```python
from build123d import *

# Parameters (mm, degrees)
SKETCH1_W               = 1200
SKETCH1_H               = 1500
BOSS_EXTRUDE1_DEPTH     = 160
BOSS_EXTRUDE2_DEPTH     = 1270
SKETCH3_W               = 125
SKETCH3_H               = 1120
CUT_EXTRUDE2_DEPTH      = 30
LPATTERN1_COUNT         = 6
LPATTERN1_PITCH         = 165
SKETCH4_W               = 125
SKETCH4_H               = 1120
CUT_EXTRUDE3_DEPTH      = 30
LPATTERN2_COUNT         = 6
LPATTERN2_PITCH         = 165
CUT_EXTRUDE5_DEPTH      = 70
CUT_EXTRUDE5_DEPTH_BACK = 3200
SKETCH5_W               = 160
SKETCH5_H               = 1200
BOSS_EXTRUDE3_DEPTH     = 40
CUT_EXTRUDE6_DEPTH      = 1622
SKETCH8_R               = 25
BOSS_EXTRUDE4_DEPTH     = 284.986135381
SKETCH10_R              = 25
BOSS_EXTRUDE5_DEPTH     = 408.541682101


with BuildPart() as part:
    # Sketch1 → Boss-Extrude1 (new body)
    with BuildSketch(Plane(origin=(0, 0, 0), x_dir=(0, 0, -1), z_dir=(1, 0, 0))):
        with Locations((564.361948956, -723.13225058)):
            Rectangle(SKETCH1_W, SKETCH1_H)
    extrude(amount=BOSS_EXTRUDE1_DEPTH)

    # Sketch2 → Boss-Extrude2 (add)
    with BuildSketch(Plane.ZY):
        Polygon((293.387128793, -77.723630642), (-775.820700233, 467.064969046), (-789.440415225, 440.33477332), (279.767413801, -104.453826367), align=None)
        Polygon((333.138052406, -383.823490794), (-736.06977662, -928.612090481), (-722.450061628, -955.342286207), (346.757767398, -410.553686519), align=None)
    extrude(amount=BOSS_EXTRUDE2_DEPTH)

    # Sketch3 → Cut-Extrude2 (cut)
    with BuildSketch(Plane(origin=(0, -466.202007743, 237.541787551), x_dir=(-1, 0, 0), z_dir=(0, -0.8910065241883673, 0.45399049973954775))):
        with Locations((1167.066310977, 477.424040248)):
            Rectangle(SKETCH3_W, SKETCH3_H)
    cut_extrude2 = extrude(amount=-CUT_EXTRUDE2_DEPTH, mode=Mode.SUBTRACT)

    # LPattern1: Cut-Extrude2 ×6
    with Locations(*[(i * LPATTERN1_PITCH, 0, 0) for i in range(1, LPATTERN1_COUNT)]):
        add(cut_extrude2, mode=Mode.SUBTRACT)

    # Sketch4 → Cut-Extrude3 (cut)
    with BuildSketch(Plane(origin=(0, 30.243173593, 15.409666619), x_dir=(-1, 0, 0), z_dir=(0, -0.891006524188367, -0.4539904997395487))):
        with Locations((1167.5, 303.304364216)):
            Rectangle(SKETCH4_W, SKETCH4_H)
    cut_extrude3 = extrude(amount=-CUT_EXTRUDE3_DEPTH, mode=Mode.SUBTRACT)

    # LPattern2: Cut-Extrude3 ×6
    with Locations(*[(i * LPATTERN2_PITCH, 0, 0) for i in range(1, LPATTERN2_COUNT)]):
        add(cut_extrude3, mode=Mode.SUBTRACT)

    # Sketch5 → Cut-Extrude5 (cut, two sides: drawn at the far end of the back side and taken through both)
    with BuildSketch(Plane(origin=(0, 26.86774942, 0), x_dir=(1, 0, 0), z_dir=(0, 1, 0)).offset(-CUT_EXTRUDE5_DEPTH_BACK)):
        with Locations((80, 564.361948956)):
            Rectangle(SKETCH5_W, SKETCH5_H)
    extrude(amount=CUT_EXTRUDE5_DEPTH + CUT_EXTRUDE5_DEPTH_BACK, mode=Mode.SUBTRACT)


with BuildPart() as cut_extrude5_piece_1:
    # of the separate pieces the step leaves, piece 1, a body of its own (cut_extrude5_pieces)
    add(part.part.solids().sort_by_distance((0, -104.453826367, 279.767413801))[0])



with BuildPart() as cut_extrude5_piece_2:
    # of the separate pieces the step leaves, piece 2, a body of its own (cut_extrude5_pieces)
    add(part.part.solids().sort_by_distance((0, -410.553686519, 346.757767398))[0])


with BuildPart() as cut_extrude5_piece_1_1:
    add(cut_extrude5_piece_1.part)

    add(cut_extrude5_piece_2.part)  # Boss-Extrude3 merges Cut-Extrude5 piece 2
    # Sketch6 → Boss-Extrude3 (add)
    with BuildSketch(Plane(origin=(0, 0, 0), x_dir=(0, 0, -1), z_dir=(1, 0, 0))):
        Polygon((-293.387128793, -77.723630642), (-346.757767398, -410.553686519), (722.450061628, -955.342286207), (775.820700233, 467.064969046), align=None)
    extrude(amount=BOSS_EXTRUDE3_DEPTH)

    # Sketch7 → Cut-Extrude6 (cut)
    with BuildSketch(Plane(origin=(40, 0, 0), x_dir=(0, 0, -1), z_dir=(1, 0, 0))):
        Polygon((779.00615654, 352.336895643), (771.36995873, 348.446058521), (722.450061628, -955.342286207), (-346.757767398, -410.553686519), (-313.704524727, -204.427005397), (-484.232359842, -291.315277235), (-228.557425004, -1565.861378417), (1566.457503136, -862.127788671), align=None)
        Polygon((771.36995873, 348.446058521), (-13.619714992, -51.52615783), (-313.704524727, -204.427005397), (-346.757767398, -410.553686519), (722.450061628, -955.342286207), align=None)
    extrude(amount=-CUT_EXTRUDE6_DEPTH, mode=Mode.SUBTRACT)

    # Sketch8 → Boss-Extrude4 (add)
    with BuildSketch(Plane(origin=(40, 0, 0), x_dir=(0, 0, -1), z_dir=(1, 0, 0))):
        with Locations(Location((-198.070529097, -84.596305771, 0), (0, 0, 180))):
            Circle(SKETCH8_R)
        with Locations(Location((678.163657159, 359.269351402, 0), (0, 0, 180))):
            Circle(SKETCH8_R)
    extrude(amount=BOSS_EXTRUDE4_DEPTH)

    # Sketch10 → Boss-Extrude5 (add)
    with BuildSketch(Plane.ZY.offset(1270)):
        with Locations(Location((-716.617969304, 403.229883829, 0), (0, 0, 153))):
            Circle(SKETCH10_R)
        with Locations(Location((171.176211965, -49.123845441, 0), (0, 0, 153))):
            Circle(SKETCH10_R)
    extrude(amount=BOSS_EXTRUDE5_DEPTH)


solid = cut_extrude5_piece_1_1.part
```
Model file for the job. Use its own axes, mm. A direction names the side the tool comes from. Coordinates: 2 decimals unless noted, no trailing zeros. Order: outer loops, then holes, each group sorted by start corner. A loop starts at its lowest first (then second) coordinate and runs counter-clockwise, first axis right, second up. Notation, with made-up numbers: (77.25, 82) - (132.25, 82) arc R8 cw to (132.25, 95) - close; hole circle Ø6 at (42, 55.5). An arc over 180 degrees is marked (long way). Return JSON: item names as keys, results as strings. Group by question number.
1) Probe line 1 (Z direction, x = -61, y = 106); line 2 (Y direction, x = 160.5, z = 209.5); line 3 (Y direction, x = -221.5, z = -625). List the from-to ranges inside material, lowest first. Write a range as from..to.
2) Saw through at B-B, the plane y = 216.5. Count the separate pieces of the cut face and the enclosed holes in it, plus the area to 3 significant figures.
3) Saw through at D-D, the plane x = -250.5. Write the cut outline in (y, z), plus the area to 3 significant figures.
4) Saw through at A-A, the plane x = -1029. Write the cut outline in (y, z).
5) Tool access for faces 1 (the cylindrical face through (-1471.41, -44.58, 195.76)), 2 (the flat face through (19.72, -140.188, 303.404)), 3 (the cylindrical face through (180.498, -92.106, 221.916)), 4 (the flat face through (19.72, 406.925, -773.564)), 5 (the flat face through (-1270, -58, 167)): list every direction of +Z, -Z, +X, -X, +Y, -Y with a clear straight run to the whole face (end or side of a thin tool).
6) Mould opens along X. For faces 6 (the cylindrical face through (180.498, 334.482, -681.418)), 7 (the flat face through (-570, 178, -241)), 8 (the flat face through (-1678.542, -50, 171)) say: released by +X, released by -X, zero draft, split by the parting line, or undercut.
7) Flat gauge pins, fed straight in: P1, Ø1.5, axis at x = -1192.5, y = -61, coming from the +Z side; P2, Ø18, axis at y = 402, z = -725.5, coming from the +X side; P3, Ø1.5, axis at x = -139.5, z = -114.5, coming from the -Y side. Where does each tip first touch, or does it go through?
Values found:
{
 "1": {"line 1": "z = -133.27..-67.19", "line 2": "y = -106.83..-62.36", "line 3": "y = 356.55..390.22"},
 "2": {"separate pieces": "7", "enclosed holes": "0", "area": "43,500 mm²"},
 "3": {"outline": "(-104.45, 279.77) - (440.33, -789.44) - (467.06, -775.82) - (-77.72, 293.39) - close", "area": "36,000 mm²"},
 "4": {"outline": "(-104.45, 279.77) - (-86.29, 244.13) - (-59.56, 257.75) - (-77.72, 293.39) - close; (422.18, -753.8) - (440.33, -789.44) - (467.06, -775.82) - (448.91, -740.18) - close"},
 "5": {"face 1": "-X", "face 2": "+Z, +X, -X, +Y", "face 3": "+X", "face 4": "-Z, +X, -Y", "face 5": "-Z, -Y"},
 "6": {"face 6": "zero draft", "face 7": "undercut", "face 8": "released by -X"},
 "7": {"P1": "stops at z = 262.04", "P2": "stops at x = 40", "P3": "stops at y = 96.05"}
}
